Geometry check sheet. Reference: drawing and pictorial views, mm from the part's lowest x, y, z. A direction names the side the tool comes from. Round coordinates to 2 decimals unless told otherwise and drop trailing zeros. Order: outer loops, then holes, each group sorted by start corner. A loop starts at its lowest first (then second) coordinate and runs counter-clockwise, first axis right, second up.
(1) Cross-section at A-A on y = 31. Enter the section's corners in (x, z), and give its area (3 significant figures).
(2) Cross-section at C-C on z = 7.75. Enter the section's corners in (x, y).
(3) Cross-section at D-D on x = 45.5. Enter the section's corners in (y, z), and give its area (3 significant figures).
(4) Set-up check for the marked faces 1 and 2: record each of +Z, -Z, +X, -X, +Y, -Y from which the full face is reachable in a straight line by a thin tool's end or side.
(5) Draft check along Y on the marked faces 3, 4, 5 and 6. Enter one of: pulls with the +Y half, pulls with the -Y half, needs draft (parallel to the pull), parting line crosses it, or undercut.
(6) Gauge pin test, flat ends, axial feed: P1, Ø24.5, axis at x = 26, y = 28, coming from the +Z side; P2, Ø4, axis at x = 24.5, z = 3.5, coming from the +Y side; P3, Ø13, axis at x = 31, y = 31, coming from the +Z side; P4, Ø2, axis at x = 32, z = 7, coming from the -Y side. Record the tip position at first contact, or that the pin passes through.
(7) Thickness scan on L1, parallel to Y at x = 31, z = 0.9; L2, parallel to Z at x = 24, y = 3; L3, parallel to Y at x = 33.5, z = 3.75. Record the ranges inside material, lowest first.
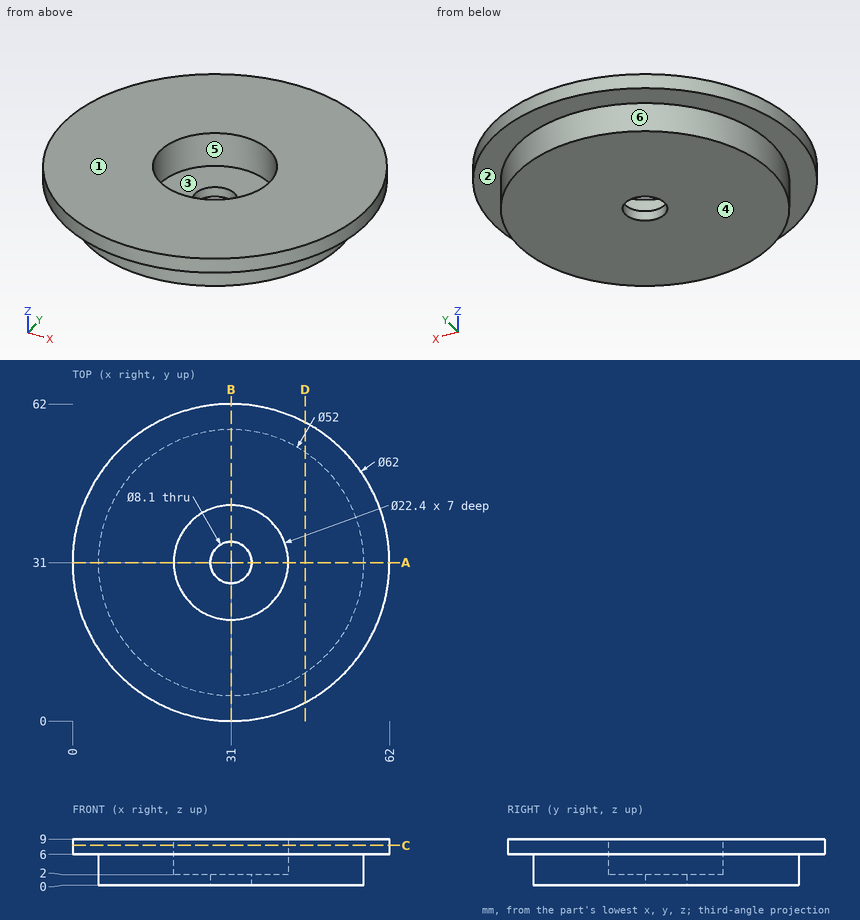
Found:
1. outline: (0, 6) - (5, 6) - (5, 0) - (26.95, 0) - (26.95, 2) - (19.8, 2) - (19.8, 9) - (0, 9) - close; (35.05, 0) - (57, 0) - (57, 6) - (62, 6) - (62, 9) - (42.2, 9) - (42.2, 2) - (35.05, 2) - close
1. area: 325 mm2
2. outline: circle Ø62 at (31, 31); hole circle Ø22.4 at (31, 31)
3. outline: (3.6, 6) - (9.42, 6) - (9.42, 0) - (52.58, 0) - (52.58, 6) - (58.4, 6) - (58.4, 9) - (3.6, 9) - close
3. area: 423 mm2
4. face 1: +Z, +X, -X, +Y, -Y
4. face 2: -Z
5. face 3: undercut
5. face 4: needs draft
5. face 5: undercut
5. face 6: parting line crosses it
6. P1: stops at z = 9
6. P2: stops at y = 56.61
6. P3: stops at z = 2
6. P4: stops at y = 0
7. L1: y = 5 to 26.95, 35.05 to 57
7. L2: z = 6 to 9
7. L3: y = 5.12 to 20.08, 41.92 to 56.88
